```python
from build123d import *

# Parameters (mm, degrees)
SKETCH2_R           = 1.190625
BOSS_EXTRUDE2_DEPTH = 1.5875
SKETCH6_R           = 1.5875
BOSS_EXTRUDE5_DEPTH = 19.05
SKETCH7_R           = 4.7625
BOSS_EXTRUDE6_DEPTH = 12.7


with BuildPart() as part:
    # Sketch2 → Boss-Extrude2 (new body, symmetric)
    with BuildSketch(Plane.XY):
        with BuildLine():
            Line((-2.667, 3.175), (-1.5875, 3.175))
            Line((-1.5875, 3.175), (1.5875, 3.175))
            Line((1.5875, 3.175), (2.667, 3.175))
            ThreePointArc((2.667, 3.175), (3.026210245, 3.026210245), (3.175, 2.667))
            Line((3.175, 2.667), (3.175, -2.667))
            ThreePointArc((3.175, -2.667), (3.026210245, -3.026210245), (2.667, -3.175))
            Line((2.667, -3.175), (-2.667, -3.175))
            ThreePointArc((-2.667, -3.175), (-3.026210245, -3.026210245), (-3.175, -2.667))
            Line((-3.175, -2.667), (-3.175, 2.667))
            ThreePointArc((-3.175, 2.667), (-3.026210245, 3.026210245), (-2.667, 3.175))
        make_face()
        Circle(SKETCH2_R, mode=Mode.SUBTRACT)
    extrude(amount=BOSS_EXTRUDE2_DEPTH, both=True)

    # Sketch6 → Boss-Extrude5 (add)
    with BuildSketch(Plane(origin=(0, 3.175, 0), x_dir=(1, 0, 0), z_dir=(0, 1, 0))):
        Circle(SKETCH6_R)
    extrude(amount=BOSS_EXTRUDE5_DEPTH)

    # Sketch7 → Boss-Extrude6 (add)
    with BuildSketch(Plane(origin=(0, 22.225, 0), x_dir=(1, 0, 0), z_dir=(0, 1, 0))):
        Circle(SKETCH7_R)
    extrude(amount=BOSS_EXTRUDE6_DEPTH)


solid = part.part
```
Here's how the part is built. I have some questions about the finished solid (model axes, mm). A direction names the side the tool comes from. Coordinates: 2 decimals unless noted, no trailing zeros. Write each loop counter-clockwise with the first axis right and the second up, starting at its lowest first coordinate (ties: lowest second). Pieces come first, ordered by that corner, then holes. Notation, with made-up numbers: (66, 57.5) -> (102, 57.5) arc R14 ccw to (102, 61.5) -> close; hole circle Ø3 at (-39, 45.5). An arc over 180 degrees is marked (long way). Use a Markdown table: item, result. Add a question column.
(1) If we section it at B-B, the plane z = 0: Write out the boundary of the cut face in (x, y) (1 decimal), and give its area (3 significant figures).
(2) I'm going to push flat-ended pins straight in: P1, Ø1, axis at x = 0.5, y = 7, coming from the -Z side; P2, Ø3.5, axis at y = 0, z = 0, coming from the +X side (3 decimals); P3, Ø2, axis at x = -3, y = 11, coming from the +Z side; P4, Ø1, axis at y = 1, z = -0.5, coming from the -X side (3 decimals). Where does each tip first touch, or does it pass through?
(3) For faces 1 (the flat face through (3.175, 0, 0)), 2 (the flat face through (2, 22.225, 0)), 3 (the flat face through (-1.4, 0, -1.588)), which set-ups out of +Z, -Z, +X, -X, +Y, -Y let a thin tool reach every point of the face, with its end or its side?
(4) Please list where these lines run through material, in increasing order: line 1 (Y direction, x = 0, z = -0.55) (3 decimals); line 2 (Y direction, x = -2.5, z = 0.5) (3 decimals); line 3 (Y direction, x = -4.25, z = 1) (3 decimals).
(5) If we section it at A-A, the plane y = 0: Write out the boundary of the cut face in (x, z) (1 decimal), and give its area (3 significant figures).
(6) We'd pull the mould along X, two halves only. Please class faces 4 (the cylindrical face through (-0.945, -0.724, -0.022)), 5 (the flat face through (-3.175, 0, 0)), 6 (the flat face through (2, 3.175, 0)), 7 (the cylindrical face through (-0.34, 12.57, 1.55)): +X half, -X half, draft (parallel to the pull), parting line (faces both ways), or undercut.
(7) If we section it at D-D, the plane y = 16: Write out the boundary of the cut face in (x, z) (1 decimal), and give its area (3 significant figures).
Outcome:
| question | item | result |
|---|---|---|
| 1 | outline | (-4.8, 22.2) -> (-1.6, 22.2) -> (-1.6, 3.2) -> (-2.7, 3.2) arc R0.5 ccw to (-3.2, 2.7) -> (-3.2, -2.7) arc R0.5 ccw to (-2.7, -3.2) -> (2.7, -3.2) arc R0.5 ccw to (3.2, -2.7) -> (3.2, 2.7) arc R0.5 ccw to (2.7, 3.2) -> (1.6, 3.2) -> (1.6, 22.2) -> (4.8, 22.2) -> (4.8, 34.9) -> (-4.8, 34.9) -> close; hole circle Ø2.4 at (0, 0) |
| 1 | area | 217 mm^2 |
| 2 | P1 | stops at z = -1.59 |
| 2 | P2 | stops at x = 3.175 |
| 2 | P3 | passes through |
| 2 | P4 | stops at x = -3.175 |
| 3 | face 1 | +Z, -Z, +X, -Y |
| 3 | face 2 | none |
| 3 | face 3 | -Z, +X, -X, -Y |
| 4 | line 1 | y = -3.175 to -1.191, 1.191 to 34.925 |
| 4 | line 2 | y = -3.175 to 3.175, 22.225 to 34.925 |
| 4 | line 3 | y = 22.225 to 34.925 |
| 5 | outline | (-3.2, -1.6) -> (-1.2, -1.6) -> (-1.2, 1.6) -> (-3.2, 1.6) -> close; (1.2, -1.6) -> (3.2, -1.6) -> (3.2, 1.6) -> (1.2, 1.6) -> close |
| 5 | area | 12.6 mm^2 |
| 6 | face 4 | undercut |
| 6 | face 5 | -X half |
| 6 | face 6 | draft |
| 6 | face 7 | parting line |
| 7 | outline | circle Ø3.2 at (0, 0) |
| 7 | area | 7.92 mm^2 |
